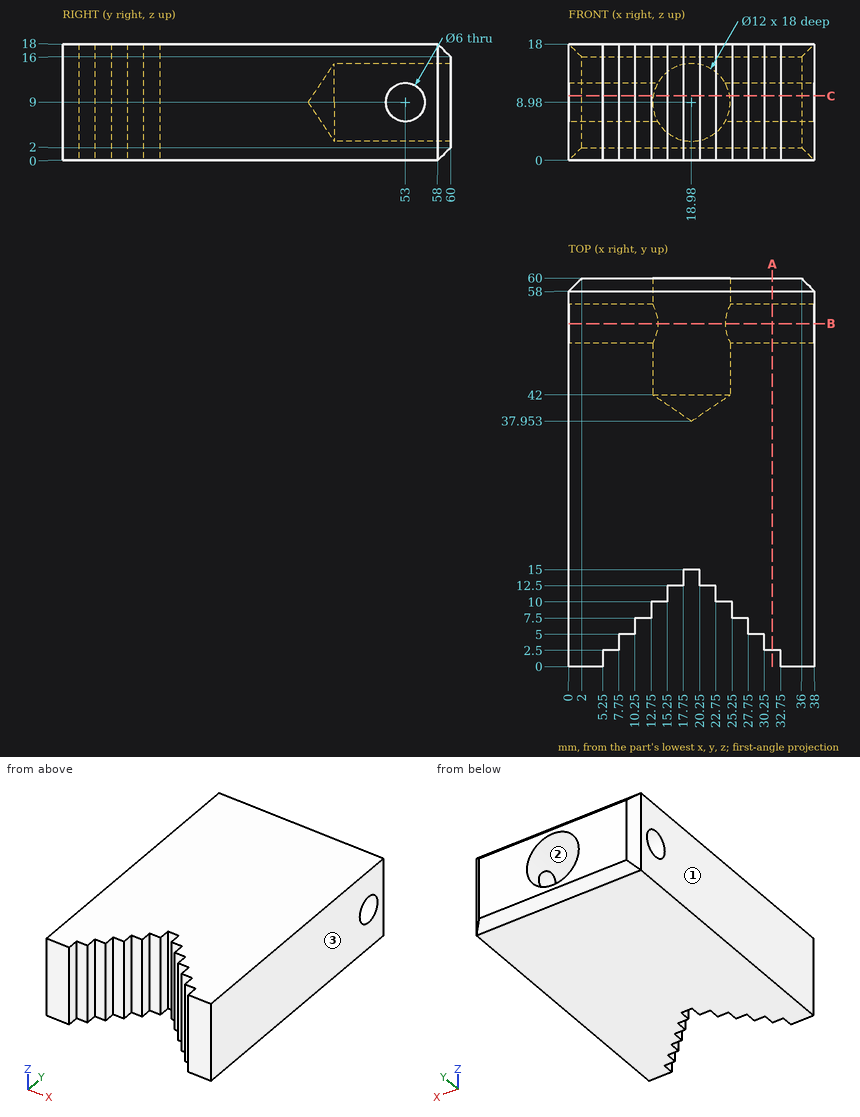
Input: dimensioned drawing with shaded views. Units: mm. Origin: part minimum x, y, z. Round coordinates to 2 decimals unless told otherwise and drop trailing zeros. Loops run counter-clockwise (first coordinate to the right, second up) from the corner with the lowest first, then second, coordinate; pieces in that order, holes last.
1) Section query C-C on z = 10. Count the separate pieces of the cut face and the enclosed holes in it, plus the area to 3 significant figures.
Ans:
separate pieces: 3
enclosed holes: 0
area: 1,670 mm2
2) Section query B-B on y = 53. Return the cut outline in (x, z) (1 decimal).
Ans:
outline: (0, 0) - (38, 0) - (38, 6) - (24.2, 6) arc R6 cw to (13.8, 6) - (0, 6) - close; (0, 12) - (13.8, 12) arc R6 cw to (24.2, 12) - (38, 12) - (38, 18) - (0, 18) - close
3) Section query A-A on x = 31.5. Return the cut outline in (y, z).
Ans:
outline: (2.5, 0) - (58, 0) - (60, 2) - (60, 16) - (58, 18) - (2.5, 18) - close; hole circle Ø6 at (53, 9)
4) Pull-direction query (X, two-part tool) for the marked faces 1, 2 and 3; classes: released by +X, released by -X, zero draft, split by the parting line, or undercut.
Ans:
face 1: released by -X
face 2: undercut
face 3: released by +X
5) Pin query (flat end, axial travel): pin 1 (1.2 mm diameter, centred on x = 6.5, z = 6.5, fed in from -Y); pin 2 (0.8 mm diameter, centred on x = 29, z = 5.5, fed in from -Y); pin 3 (0.8 mm diameter, centred on x = 21, z = 13, fed in from -Y). Return the tip coordinate at first contact, or that it passes through.
Ans:
pin 1: stops at y = 2.5
pin 2: stops at y = 5
pin 3: stops at y = 12.5
6) Material intervals for line 1 (Z direction, x = 29.5, y = 53); line 2 (X direction, y = 5.5, z = 15.25); line 3 (Z direction, x = 9.5, y = 52), sorted ascending.
Ans:
line 1: z = 0 to 6, 12 to 18
line 2: x = 0 to 10.25, 27.75 to 38
line 3: z = 0 to 6.17, 11.83 to 18
